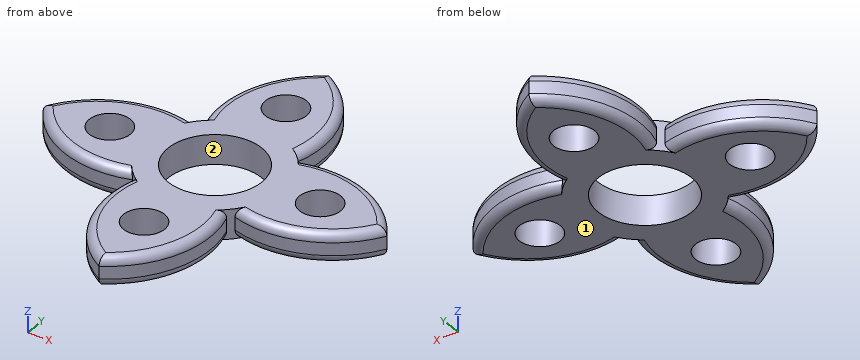
from build123d import *

# Parameters (mm, degrees)
F0_R     = 11.15
F0_R_2   = 4.9
F0_R_3   = 7.9261864564
F1_DEPTH = 7
F2_R     = 2


with BuildPart() as f1:
    # F0 (on Top) → F1 (new body)
    with BuildSketch(Plane.XY):
        with BuildLine():
            ThreePointArc((12.2001039663, -11.0155566574), (15.3414775392, -5.9011941313), (16.4373059003, 0))
            ThreePointArc((16.4373059003, 0), (15.3414775392, 5.9011941313), (12.2001039663, 11.0155566574))
            ThreePointArc((12.2001039663, 11.0155566574), (11.6229304666, 11.6229304666), (11.0155566574, 12.2001039663))
            ThreePointArc((11.0155566574, 12.2001039663), (0, 16.4373059003), (-11.0155566574, 12.2001039663))
            ThreePointArc((-11.0155566574, 12.2001039663), (-11.6229304666, 11.6229304666), (-12.2001039663, 11.0155566574))
            ThreePointArc((-12.2001039663, 11.0155566574), (-16.4373059003, 0), (-12.2001039663, -11.0155566574))
            ThreePointArc((-12.2001039663, -11.0155566574), (-11.6229304666, -11.6229304666), (-11.0155566574, -12.2001039663))
            ThreePointArc((-11.0155566574, -12.2001039663), (0, -16.4373059003), (11.0155566574, -12.2001039663))
            ThreePointArc((11.0155566574, -12.2001039663), (11.6229304666, -11.6229304666), (12.2001039663, -11.0155566574))
        make_face()
        Circle(F0_R, mode=Mode.SUBTRACT)
        with BuildLine():
            ThreePointArc((-11.0155566574, 12.2001039663), (0, 16.4373059003), (11.0155566574, 12.2001039663))
            ThreePointArc((11.0155566574, 12.2001039663), (10.5712674009, 28.4766709057), (0, 40.8610291779))
            ThreePointArc((0, 40.8610291779), (-10.5712674009, 28.4766709057), (-11.0155566574, 12.2001039663))
        make_face()
        with Locations((0, 25)):
            Circle(F0_R_2, mode=Mode.SUBTRACT)
        with BuildLine():
            ThreePointArc((0, -40.8610291779), (10.5712674009, -28.4766709057), (11.0155566574, -12.2001039663))
            ThreePointArc((11.0155566574, -12.2001039663), (0, -16.4373059003), (-11.0155566574, -12.2001039663))
            ThreePointArc((-11.0155566574, -12.2001039663), (-10.5712674009, -28.4766709057), (0, -40.8610291779))
        make_face()
        with Locations((0, -25)):
            Circle(F0_R_2, mode=Mode.SUBTRACT)
        with BuildLine():
            ThreePointArc((12.2001039663, 11.0155566574), (15.3414775392, 5.9011941313), (16.4373059003, 0))
            ThreePointArc((16.4373059003, 0), (15.3414775392, -5.9011941313), (12.2001039663, -11.0155566574))
            ThreePointArc((12.2001039663, -11.0155566574), (28.4766709057, -10.5712674009), (40.8610291779, 0))
            ThreePointArc((40.8610291779, 0), (28.4766709057, 10.5712674009), (12.2001039663, 11.0155566574))
        make_face()
        with Locations((25, 0)):
            Circle(F0_R_3, mode=Mode.SUBTRACT)
        with BuildLine():
            ThreePointArc((-12.2001039663, -11.0155566574), (-16.4373059003, 0), (-12.2001039663, 11.0155566574))
            ThreePointArc((-12.2001039663, 11.0155566574), (-28.4766709057, 10.5712674009), (-40.8610291779, 0))
            ThreePointArc((-40.8610291779, 0), (-28.4766709057, -10.5712674009), (-12.2001039663, -11.0155566574))
        make_face()
        with Locations((-25, 0)):
            Circle(F0_R_2, mode=Mode.SUBTRACT)
        with Locations((25, 0)):
            Circle(F0_R_3)
        with Locations((25, 0)):
            Circle(F0_R_2, mode=Mode.SUBTRACT)
    extrude(amount=F1_DEPTH)

    # F2
    f2_edges = [f1.edges().sort_by_distance(p)[0] for p in [
        (-10.571267, 28.476671, 7),
        (10.571267, 28.476671, 7),
        (28.476671, -10.571267, 7),
        (28.476671, 10.571267, 7),
        (10.571267, -28.476671, 7),
        (-10.571267, -28.476671, 7),
        (-28.476671, -10.571267, 7),
        (-28.476671, 10.571267, 7),
        (10.571267, 28.476671, 0),
        (-10.571267, 28.476671, 0),
        (-28.476671, 10.571267, 0),
        (-28.476671, -10.571267, 0),
        (10.571267, -28.476671, 0),
        (-10.571267, -28.476671, 0),
        (28.476671, 10.571267, 0),
        (28.476671, -10.571267, 0),
    ]]
    fillet(f2_edges, radius=F2_R)


solid = f1.part
Verification items for the finished model (mm, model axes). Face numbers are marked on the shaded views. Coordinates: 2 decimals unless noted, no trailing zeros. Loops run counter-clockwise (first coordinate to the right, second up) from the corner with the lowest first, then second, coordinate; pieces in that order, holes last. Notation, with made-up numbers: (-23.75, 8.5) -> (18.25, 8.5) arc R19 ccw to (18.25, 41.5) -> close; hole circle Ø7 at (-18.5, 68). An arc over 180 degrees is marked (long way). Write each question's results on one line, items separated by ' | '.
Item 1: Gauge pin test, flat ends, axial feed: pin 1 (3 mm diameter, centred on y = 10, z = 2.5, fed in from -X) (3 decimals); pin 2 (1 mm diameter, centred on y = -24.5, z = 6, fed in from -X); pin 3 (4 mm diameter, centred on x = 5, z = 1.5, fed in from -Y). Record the tip position at first contact, or that the pin passes through.
Found:
pin 1: stops at x = -32.635 | pin 2: stops at x = -11.69 | pin 3: stops at y = -38.78
Item 2: Section check B-B, the plane y = -3. Count the separate pieces of the cut face and the enclosed holes in it, plus the area to 3 significant figures.
Found:
separate pieces: 4 | enclosed holes: 0 | area: 280 mm2
Item 3: Section check A-A, the plane z = 3.25. Enter the section's corners in (x, y).
Found:
outline: (-40.86, 0) arc R24.44 ccw to (-12.2, -11.02) arc R16.44 ccw to (-11.02, -12.2) arc R24.44 ccw to (0, -40.86) arc R24.44 ccw to (11.02, -12.2) arc R16.44 ccw to (12.2, -11.02) arc R24.44 ccw to (40.86, 0) arc R24.44 ccw to (12.2, 11.02) arc R16.44 ccw to (11.02, 12.2) arc R24.44 ccw to (0, 40.86) arc R24.44 ccw to (-11.02, 12.2) arc R16.44 ccw to (-12.2, 11.02) arc R24.44 ccw to start; hole circle Ø9.8 at (-25, 0); hole circle Ø22.3 at (0, 0); hole circle Ø9.8 at (0, -25); hole circle Ø9.8 at (0, 25); hole circle Ø9.8 at (25, 0)
Item 4: Mould release check, pull along X, two halves, no side actions. Record for the marked faces 1 and 2: +X half, -X half, draft (parallel to the pull), parting line (faces both ways), or undercut.
Found:
face 1: draft | face 2: undercut
Item 5: Material ranges on L1, parallel to Y at x = 0, z = 4.5; L2, parallel to X at y = -2, z = 1.5; L3, parallel to Y at x = 0.5, z = 3.25, recorded low to high.
Found:
L1: y = -40.86 to -29.9, -20.1 to -11.15, 11.15 to 20.1, 29.9 to 40.86 | L2: x = -39.49 to -29.47, -20.53 to -10.97, 10.97 to 20.53, 29.47 to 39.49 | L3: y = -40.56 to -29.87, -20.13 to -11.14, 11.14 to 20.13, 29.87 to 40.56
